from build123d import *

# Parameters (mm, degrees)
F1_DEPTH     = 101.6
F2_T1_DEPTH  = 101.6
F2_T3_DEPTH  = 24.6862719756
F2_T5_DEPTH  = 127
F2_T7_DEPTH  = 94.8975325807
F2_T9_DEPTH  = 67.8662719756
F2_T11_DEPTH = 109.22
F2_T13_DEPTH = 100.4137670475
F2_T15_DEPTH = 50.0862719756
F2_S19_W     = 5.1816
F2_S19_H     = 5.1816
F2_T20_DEPTH = 5.1816
F2_T24_ANGLE = 90
F2_T26_ANGLE = 90
F3_T1_DEPTH  = 82.6337670475
F3_T3_DEPTH  = 15.24
F3_S7_W      = 5.08
F3_S7_H      = 5.08
F3_T8_DEPTH  = 5.08
F3_S13_W     = 5.08
F3_S13_H     = 5.08
F3_T14_DEPTH = 5.08
F3_T18_ANGLE = 89.9999999979


# Not quite as in the source:
# - a fillet or chamfer that OpenCascade refuses, or shapes differently, is made with other operations: its cross-section is extruded or revolved along the edge and cut away or added


with BuildPart() as f1:
    # F0 (on Front) → F1 (new body)
    with BuildSketch(Plane.XZ):
        Polygon((-47.2256254691, 25.4), (-128.5056254691, 25.4), (-128.5056254691, 0), (-41.2280928884, 0), (-41.2280928884, -17.0662719756), (-35.7118584216, -17.0662719756), (-35.7118584216, 25.4), align=None)
    extrude(amount=F1_DEPTH)

    # F2: fillet of radius 5.08 on 11 edges, made by hand

    # F2_s2 → F2_t1 (join)
    with BuildSketch(Plane.XZ):
        with BuildLine():
            ThreePointArc((-41.2280928884, -5.08), (-42.71599044, -1.4878975516), (-46.3080928884, 0))
            Line((-46.3080928884, 0), (-41.2280928884, 0))
            Line((-41.2280928884, 0), (-41.2280928884, -5.08))
        make_face()
    extrude(amount=F2_T1_DEPTH)

    # F2_s4 → F2_t3 (cut)
    with BuildSketch(Plane.XY.offset(-29.7662719756)):
        with BuildLine():
            ThreePointArc((-36.1480928884, 0), (-39.7401953368, -1.4878975516), (-41.2280928884, -5.08))
            Line((-41.2280928884, -5.08), (-41.2280928884, 0))
            Line((-41.2280928884, 0), (-36.1480928884, 0))
        make_face()
        with BuildLine():
            ThreePointArc((-36.1480928884, -101.6), (-39.7401953368, -100.1121024484), (-41.2280928884, -96.52))
            Line((-41.2280928884, -96.52), (-41.2280928884, -101.6))
            Line((-41.2280928884, -101.6), (-36.1480928884, -101.6))
        make_face()
    extrude(amount=F2_T3_DEPTH, mode=Mode.SUBTRACT)

    # F2_s6 → F2_t5 (cut)
    with BuildSketch(Plane.XZ.offset(-12.7)):
        with BuildLine():
            ThreePointArc((-128.5056254691, 5.08), (-127.0177279175, 1.4878975516), (-123.4256254691, 0))
            Line((-123.4256254691, 0), (-128.5056254691, 0))
            Line((-128.5056254691, 0), (-128.5056254691, 5.08))
        make_face()
        with BuildLine():
            ThreePointArc((-123.4256254691, 25.4), (-127.0177279175, 23.9121024484), (-128.5056254691, 20.32))
            Line((-128.5056254691, 20.32), (-128.5056254691, 25.4))
            Line((-128.5056254691, 25.4), (-123.4256254691, 25.4))
        make_face()
    extrude(amount=F2_T5_DEPTH, mode=Mode.SUBTRACT)

    # F2_s8 → F2_t7 (cut)
    with BuildSketch(Plane.YZ.offset(-141.2056254691)):
        with BuildLine():
            ThreePointArc((0, 5.08), (-1.4878975516, 1.4878975516), (-5.08, 0))
            Line((-5.08, 0), (0, 0))
            Line((0, 0), (0, 5.08))
        make_face()
        with BuildLine():
            ThreePointArc((-101.6, 5.08), (-100.1121024484, 1.4878975516), (-96.52, 0))
            Line((-96.52, 0), (-101.6, 0))
            Line((-101.6, 0), (-101.6, 5.08))
        make_face()
    extrude(amount=F2_T7_DEPTH, mode=Mode.SUBTRACT)

    # F2_s10 → F2_t9 (cut)
    with BuildSketch(Plane.XY.offset(-29.7662719756)):
        with BuildLine():
            ThreePointArc((-35.7118584216, -96.52), (-37.1997559731, -100.1121024484), (-40.7918584216, -101.6))
            Line((-40.7918584216, -101.6), (-35.7118584216, -101.6))
            Line((-35.7118584216, -101.6), (-35.7118584216, -96.52))
        make_face()
    extrude(amount=F2_T9_DEPTH, mode=Mode.SUBTRACT)

    # F2_s12 → F2_t11 (cut)
    with BuildSketch(Plane.XZ.offset(5.08)):
        with BuildLine():
            ThreePointArc((-40.7918584216, 25.4), (-37.1997559731, 23.9121024484), (-35.7118584216, 20.32))
            Line((-35.7118584216, 20.32), (-35.7118584216, 25.4))
            Line((-35.7118584216, 25.4), (-40.7918584216, 25.4))
        make_face()
    extrude(amount=F2_T11_DEPTH, mode=Mode.SUBTRACT)

    # F2_s14 → F2_t13 (cut)
    with BuildSketch(Plane.YZ.offset(-141.2056254691)):
        with BuildLine():
            ThreePointArc((-5.08, 25.4), (-1.4878975516, 23.9121024484), (0, 20.32))
            Line((0, 20.32), (0, 25.4))
            Line((0, 25.4), (-5.08, 25.4))
        make_face()
    extrude(amount=F2_T13_DEPTH, mode=Mode.SUBTRACT)

    # F2_s16 → F2_t15 (cut)
    with BuildSketch(Plane.XY.offset(-29.7662719756)):
        with BuildLine():
            ThreePointArc((-40.7918584216, 0), (-37.1997559731, -1.4878975516), (-35.7118584216, -5.08))
            Line((-35.7118584216, -5.08), (-35.7118584216, 0))
            Line((-35.7118584216, 0), (-40.7918584216, 0))
        make_face()
    extrude(amount=F2_T15_DEPTH, mode=Mode.SUBTRACT)


with BuildPart() as f2_tool18:
    # F2_s19 → F2_t20 (new body)
    with BuildSketch(Plane.XY.offset(20.32)):
        with Locations((-38.2010584216, -2.4892)):
            Rectangle(F2_S19_W, F2_S19_H)
    extrude(amount=F2_T20_DEPTH)

    # F2_s21 → F2_t22 (revolve, cut)
    with BuildSketch(Plane(origin=(-40.7918584216, -5.08, 20.32), x_dir=(-0.7071067812, -0.7071067812, 0), z_dir=(-0.7071067812, 0.7071067812, 0))):
        with BuildLine():
            ThreePointArc((0, -5.08), (5.08, 0), (0, 5.08))
            Line((0, 5.08), (0, -5.08))
        make_face()
    revolve(axis=Axis((-40.7918584216, -5.08, 20.32), (0, 0, 1)), mode=Mode.SUBTRACT)


with BuildPart() as f1_1:
    add(f1.part)

    # F2_t17: cut F2_tool18
    add(f2_tool18.part, mode=Mode.SUBTRACT)

    # F2_s23 → F2_t24 (revolve, cut)
    with BuildSketch(Plane.XY.offset(-5.08)):
        with BuildLine():
            ThreePointArc((-36.1480928884, -101.6), (-39.7401953368, -100.1121024484), (-41.2280928884, -96.52))
            Line((-41.2280928884, -96.52), (-41.2280928884, -101.6))
            Line((-41.2280928884, -101.6), (-36.1480928884, -101.6))
        make_face()
    revolve(axis=Axis((-46.3080928884, -101.6, -5.08), (0, -1, 0)), revolution_arc=F2_T24_ANGLE, mode=Mode.SUBTRACT)

    # F2_s25 → F2_t26 (revolve, cut)
    with BuildSketch(Plane.XY.offset(-5.08)):
        with BuildLine():
            ThreePointArc((-36.1480928884, 0), (-39.7401953368, -1.4878975516), (-41.2280928884, -5.08))
            Line((-41.2280928884, -5.08), (-41.2280928884, 0))
            Line((-41.2280928884, 0), (-36.1480928884, 0))
        make_face()
    revolve(axis=Axis((-46.3080928884, 0, -5.08), (0, -1, 0)), revolution_arc=F2_T26_ANGLE, mode=Mode.SUBTRACT)

    # F3: fillet of radius 5.08 on 3 edges, made by hand

    # F3_s2 → F3_t1 (cut)
    with BuildSketch(Plane.YZ.offset(-123.4256254691)):
        with BuildLine():
            ThreePointArc((-96.52, 25.4), (-100.1121024484, 23.9121024484), (-101.6, 20.32))
            Line((-101.6, 20.32), (-101.6, 25.4))
            Line((-101.6, 25.4), (-96.52, 25.4))
        make_face()
    extrude(amount=F3_T1_DEPTH, mode=Mode.SUBTRACT)

    # F3_s4 → F3_t3 (cut)
    with BuildSketch(Plane.XY.offset(5.08)):
        with BuildLine():
            ThreePointArc((-123.4256254691, -101.6), (-127.0177279175, -100.1121024484), (-128.5056254691, -96.52))
            Line((-128.5056254691, -96.52), (-128.5056254691, -101.6))
            Line((-128.5056254691, -101.6), (-123.4256254691, -101.6))
        make_face()
    extrude(amount=F3_T3_DEPTH, mode=Mode.SUBTRACT)


with BuildPart() as f3_tool6:
    # F3_s7 → F3_t8 (new body)
    with BuildSketch(Plane.XZ.offset(96.52)):
        with Locations((-125.9656254691, 2.54)):
            Rectangle(F3_S7_W, F3_S7_H)
    extrude(amount=F3_T8_DEPTH)

    # F3_s9 → F3_t10 (revolve, cut)
    with BuildSketch(Plane(origin=(-123.4256254691, -96.52, 5.08), x_dir=(0.7071067812, 0, 0.7071067812), z_dir=(0.7071067812, 0, -0.7071067812))):
        with BuildLine():
            ThreePointArc((0, -5.08), (5.08, 0), (0, 5.08))
            Line((0, 5.08), (0, -5.08))
        make_face()
    revolve(axis=Axis((-123.4256254691, -96.52, 5.08), (0, -1, 0)), mode=Mode.SUBTRACT)


with BuildPart() as f1_2:
    add(f1_1.part)

    # F3_t5: cut F3_tool6
    add(f3_tool6.part, mode=Mode.SUBTRACT)


with BuildPart() as f3_tool12:
    # F3_s13 → F3_t14 (new body)
    with BuildSketch(Plane.XY.offset(20.32)):
        with Locations((-38.2518584216, -99.06)):
            Rectangle(F3_S13_W, F3_S13_H)
    extrude(amount=F3_T14_DEPTH)

    # F3_s15 → F3_t16 (revolve, cut)
    with BuildSketch(Plane(origin=(-40.7918584216, -96.52, 20.32), x_dir=(-0.7071067812, 0.7071067812, 0), z_dir=(0.7071067812, 0.7071067812, 0))):
        with BuildLine():
            ThreePointArc((0, -5.08), (5.08, 0), (0, 5.08))
            Line((0, 5.08), (0, -5.08))
        make_face()
    revolve(axis=Axis((-40.7918584216, -96.52, 20.32), (0, 0, 1)), mode=Mode.SUBTRACT)


with BuildPart() as f1_3:
    add(f1_2.part)

    # F3_t11: cut F3_tool12
    add(f3_tool12.part, mode=Mode.SUBTRACT)

    # F3_s17 → F3_t18 (revolve, cut)
    with BuildSketch(Plane.XY.offset(20.3199999999)):
        with BuildLine():
            ThreePointArc((-128.5056254691, -96.52), (-127.0177279175, -100.1121024484), (-123.4256254691, -101.6))
            Line((-123.4256254691, -101.6), (-128.5056254691, -101.6))
            Line((-128.5056254691, -101.6), (-128.5056254691, -96.52))
        make_face()
    revolve(axis=Axis((-123.425625469, -101.6, 20.3199999999), (0, 1, 0)), revolution_arc=F3_T18_ANGLE, mode=Mode.SUBTRACT)


solid = f1_3.part
Work out the finished part from the listing and answer in its coordinate system (mm). A direction names the side the tool comes from. Give positions to 0.01 mm unless a question says otherwise; leave off trailing zeros. Loops run counter-clockwise (first coordinate to the right, second up) from the corner with the lowest first, then second, coordinate; pieces in that order, holes last. Notation, with made-up numbers: (60.25, 62.5) -> (109.25, 62.5) arc R20 cw to (109.25, 87.5) -> close; hole circle Ø11 at (54, 41.25). An arc over 180 degrees is marked (long way). Use a Markdown table: item, result. Add a question column.
1. Flat-ended cylindrical pins translate along their axes: pin 1 Ø5 at (x, z) = (-55, 1) entering from -Y; pin 2 Ø4 at (x, y) = (-93, -69.5) entering from -Z; pin 3 Ø3.5 at (y, z) = (-34.5, -10) entering from -X. Find the tip coordinate at first contact, or state that the pin passes through.
2. For faces 1 (the cylindrical face through (-40.464, -2.4, -11.157)), 2 (the cylindrical face through (-36.6, -99.39, 1.37)), 3 (the flat face through (-85, -50, 0)), 4 (the cylindrical face through (-85.407, -100.151, 1.528)), determine the directions among +Z, -Z, +X, -X, +Y, -Y from which every point of the face is accessible in a straight line to the end or side of a thin tool.
3. Section B-B on z = -13 is taken. Determine the outline of the cut face in (x, y).
4. Find the intervals of material crossed by probe 1 along Z at (x, y) = (-84.5, -75.5); probe 2 along X at (y, z) = (-71, -10); probe 3 along Y at (x, z) = (-69, 5), in increasing order.
5. Section C-C on x = -117.5 is taken. Determine the outline of the cut face in (y, z), and give its area (3 significant figures).
6. Section A-A on y = -23 is taken. Determine the outline of the cut face in (x, z), and give its area (3 significant figures).
Results below:
| question | item | result |
|---|---|---|
| 1 | pin 1 | stops at y = -101.35 |
| 1 | pin 2 | stops at z = 0 |
| 1 | pin 3 | stops at x = -41.23 |
| 2 | face 1 | -Z, -X, +Y |
| 2 | face 2 | +Z, -Z, +X, -Y |
| 2 | face 3 | -Z, -X, +Y, -Y |
| 2 | face 4 | -Z, -X, -Y |
| 3 | outline | (-41.23, -96.52) arc R5.08 ccw to (-38.47, -101.04) arc R5.08 ccw to (-35.71, -96.52) -> (-35.71, -5.08) arc R5.08 ccw to (-38.47, -0.56) arc R5.08 ccw to (-41.23, -5.08) -> close |
| 4 | probe 1 | z = 0 to 25.4 |
| 4 | probe 2 | x = -41.23 to -35.71 |
| 4 | probe 3 | y = -101.6 to 0 |
| 5 | outline | (-101.6, 5.08) arc R5.08 ccw to (-96.52, 0) -> (-5.08, 0) arc R5.08 ccw to (0, 5.08) -> (0, 20.32) arc R5.08 ccw to (-5.08, 25.4) -> (-96.52, 25.4) arc R5.08 ccw to (-101.6, 20.32) -> close |
| 5 | area | 2,560 mm^2 |
| 6 | outline | (-128.51, 5.08) arc R5.08 ccw to (-123.43, 0) -> (-46.31, 0) arc R5.08 cw to (-41.23, -5.08) -> (-41.23, -17.07) -> (-35.71, -17.07) -> (-35.71, 20.32) arc R5.08 ccw to (-40.79, 25.4) -> (-123.43, 25.4) arc R5.08 ccw to (-128.51, 20.32) -> close |
| 6 | area | 2,440 mm^2 |
